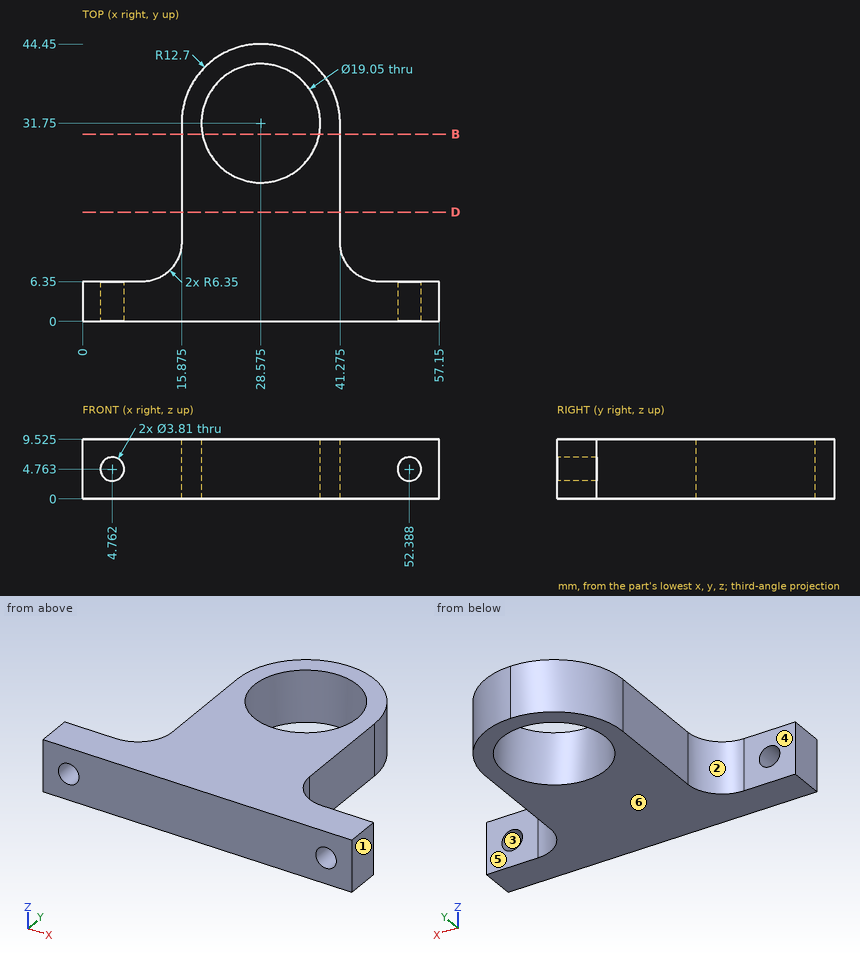
Source: three-view drawing plus pictorial views. Frame: mm from the lowest corner of the part. A direction names the side the tool comes from. Round coordinates to 2 decimals unless told otherwise and drop trailing zeros. Order: outer loops, then holes, each group sorted by start corner. A loop starts at its lowest first (then second) coordinate and runs counter-clockwise, first axis right, second up. Notation, with made-up numbers: (32.5, 26) -> (38.5, 26) arc R16 ccw to (38.5, 41) -> close; hole circle Ø1 at (59, -23). An arc over 180 degrees is marked (long way). Use one line per item in the form item = value. Start each with the question number.
1. Draft query along X for the marked faces 1, 2 and 3. Return one class per face: pulls with the +X half, pulls with the -X half, needs draft (parallel to the pull), parting line crosses it, or undercut.
2. Cut plane D-D (y = 17.5). Return the cut outline in (x, z) (1 decimal), then the cut area to 3 significant figures.
3. Reachability of the marked faces 4, 5 and 6 from +Z, -Z, +X, -X, +Y, -Y: full face, straight path, thin tool, end or side. Return the list, or none.
4. Pin query (flat end, axial travel): pin 1 Ø5 at (y, z) = (21.5, 3) entering from -X (1 decimal); pin 2 Ø3 at (x, z) = (3, 6.5) entering from +Y; pin 3 Ø3 at (y, z) = (20.5, 6.5) entering from +X (1 decimal); pin 4 Ø17 at (x, y) = (28.575, 31.75) entering from -Z. Return the tip coordinate at first contact, or that it passes through.
5. Line query: probe 1 along X at (y, z) = (5, 5); probe 2 along X at (y, z) = (26.5, 1.5) (1 decimal); probe 3 along X at (y, z) = (35.5, 2.75). Output: solid intervals per line, ascending.
6. Cut plane B-B (y = 30). Return the cut outline in (x, z) (1 decimal).
Solution:
q1.face_1 = pulls with the +X half
q1.face_2 = pulls with the -X half
q1.face_3 = undercut
q2.outline = (15.9, 0) -> (41.3, 0) -> (41.3, 9.5) -> (15.9, 9.5) -> close
q2.area = 242 mm^2
q3.face_4 = +Z, -Z, -X, +Y
q3.face_5 = +Z, -Z, +X, +Y
q3.face_6 = -Z, +X, -X, +Y, -Y
q4.pin_1 = 15.9
q4.pin_2 = 6.35
q4.pin_3 = 41.3
q4.pin_4 = through
q5.probe_1 = 0 to 2.87, 6.65 to 50.5, 54.28 to 57.15
q5.probe_2 = 15.9 to 20.6, 36.5 to 41.3
q5.probe_3 = 16.44 to 19.82, 37.33 to 40.71
q6.outline = (15.9, 0) -> (19.2, 0) -> (19.2, 9.5) -> (15.9, 9.5) -> close; (37.9, 0) -> (41.3, 0) -> (41.3, 9.5) -> (37.9, 9.5) -> close
